Here's how the part is built. I have some questions about the finished solid (model axes, mm). Face numbers are marked on the shaded views. A direction names the side the tool comes from. Coordinates: 2 decimals unless noted, no trailing zeros. Order: outer loops, then holes, each group sorted by start corner. A loop starts at its lowest first (then second) coordinate and runs counter-clockwise, first axis right, second up. Notation, with made-up numbers: M -36.5,-8 L -11.5,-8 A16 ccw -11.5,12 Z; hole C 82.5,-33.5 d3. An arc over 180 degrees is marked long. One line per question, with ' | ' between items. Start each with the question number.
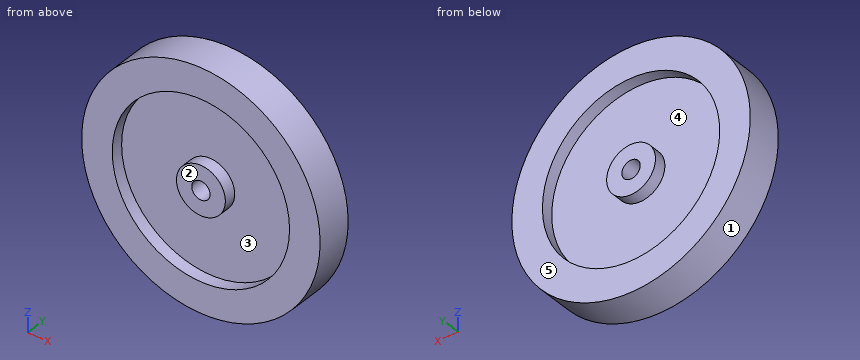
```python
from build123d import *

# Parameters (mm, degrees)
F0_R     = 4.000005
F0_R_2   = 1.499997
F1_DEPTH = 2.999994
F2_DEPTH = 2.999994
F0_R_3   = 14.499971
F3_DEPTH = 1.000001
F4_DEPTH = 1.000001
F0_R_4   = 19.499961
F5_DEPTH = 2.999994
F6_DEPTH = 2.999994


with BuildPart() as f1:
    # F0 (on Front) → F1 (new body)
    with BuildSketch(Plane.XZ):
        Circle(F0_R)
        Circle(F0_R_2, mode=Mode.SUBTRACT)
    extrude(amount=F1_DEPTH)

    # F0 (on Front) → F2 (join)
    with BuildSketch(Plane.XZ):
        Circle(F0_R)
        Circle(F0_R_2, mode=Mode.SUBTRACT)
    extrude(amount=-F2_DEPTH)

    # F0 (on Front) → F3 (join)
    with BuildSketch(Plane.XZ):
        Circle(F0_R_3)
        Circle(F0_R, mode=Mode.SUBTRACT)
    extrude(amount=F3_DEPTH)

    # F0 (on Front) → F4 (join)
    with BuildSketch(Plane.XZ):
        Circle(F0_R_3)
        Circle(F0_R, mode=Mode.SUBTRACT)
    extrude(amount=-F4_DEPTH)

    # F0 (on Front) → F5 (join)
    with BuildSketch(Plane.XZ):
        Circle(F0_R_4)
        Circle(F0_R_3, mode=Mode.SUBTRACT)
    extrude(amount=F5_DEPTH)

    # F0 (on Front) → F6 (join)
    with BuildSketch(Plane.XZ):
        Circle(F0_R_4)
        Circle(F0_R_3, mode=Mode.SUBTRACT)
    extrude(amount=-F6_DEPTH)


solid = f1.part
```
1. Will these pins go through, and if not, where does the flat tip stop? pin 1 (2 mm diameter, centred on x = -4.5, z = 9, fed in from +Y); pin 2 (1.5 mm diameter, centred on x = 4, y = -2.5, fed in from -Z); pin 3 (2.5 mm diameter, centred on x = 0, z = 0, fed in from -Y); pin 4 (5 mm diameter, centred on x = -9.5, z = 5.5, fed in from -Y).
2. Imagine slicing it at B-B (z = 0). List the corners of the cut face in (x, y) for me.
3. I need wall thicknesses on line 1 (Z direction, x = 0, y = -2.1); line 2 (Z direction, x = 8.5, y = -2.1); line 3 (Y direction, x = 11, z = -8). Which ranges of each line are inside material? Lowest first, please.
4. Imagine slicing it at C-C (y = 2.2). List the corners of the cut face in (x, z) for me, then the cut area to 3 significant figures.
5. Which directions (+Z, -Z, +X, -X, +Y, -Y) give clear straight access to the entire face, cutting with the end or side of a thin tool? Please do the marked faces 4 and 5.
6. Imagine slicing it at A-A (x = 0). List the corners of the cut face in (y, z) for me.
7. Imagine slicing it at D-D (y = 0.25). List the corners of the cut face in (x, z) for me, then the cut area to 3 significant figures.
8. We'd pull the mould along X, two halves only. Please class the marked faces 1, 2 and 3: released by +X, released by -X, zero draft, split by the parting line, or undercut.
Entries:
1) pin 1: y = 1 | pin 2: z = -19.23 | pin 3: through | pin 4: y = -1
2) outline: M -19.5,-3 L -14.5,-3 L -14.5,-1 L -4,-1 L -4,-3 L -1.5,-3 L -1.5,3 L -4,3 L -4,1 L -14.5,1 L -14.5,3 L -19.5,3 Z; M 1.5,-3 L 4,-3 L 4,-1 L 14.5,-1 L 14.5,-3 L 19.5,-3 L 19.5,3 L 14.5,3 L 14.5,1 L 4,1 L 4,3 L 1.5,3 Z
3) line 1: -19.5 to -14.5, -4 to -1.5, 1.5 to 4, 14.5 to 19.5 | line 2: -17.55 to -11.75, 11.75 to 17.55 | line 3: -1 to 1
4) outline: C 0,0 d39; C 0,0 d8; hole C 0,0 d29; hole C 0,0 d3 | area: 577 mm²
5) face 4: +Y | face 5: +Z, -Z, +X, -X, +Y
6) outline: M -3,-19.5 L 3,-19.5 L 3,-14.5 L 1,-14.5 L 1,-4 L 3,-4 L 3,-1.5 L -3,-1.5 L -3,-4 L -1,-4 L -1,-14.5 L -3,-14.5 Z; M -3,1.5 L 3,1.5 L 3,4 L 1,4 L 1,14.5 L 3,14.5 L 3,19.5 L -3,19.5 L -3,14.5 L -1,14.5 L -1,4 L -3,4 Z
7) outline: C 0,0 d39; hole C 0,0 d3 | area: 1,190 mm²
8) face 1: split by the parting line | face 2: zero draft | face 3: undercut
